```python
from build123d import *

# Parameters (mm, degrees)
SKETCH1_W           = 50
SKETCH1_H           = 80
BOSS_EXTRUDE1_DEPTH = 4.5
SKETCH2_R           = 0.5
CUT_EXTRUDE1_DEPTH  = 95.447075127
SKETCH3_W           = 2
SKETCH3_H           = 2.25
CUT_EXTRUDE2_DEPTH  = 95.447075127
SKETCH5_R           = 2.5
BOSS_EXTRUDE2_DEPTH = 2
SKETCH6_R           = 1.5
CUT_EXTRUDE3_DEPTH  = 95.563470748
FILLET1_R           = 4
SKETCH8_W           = 5.5
SKETCH8_H           = 30
CUT_EXTRUDE4_DEPTH  = 3


with BuildPart() as part:
    # Sketch1 → Boss-Extrude1 (new body)
    with BuildSketch(Plane(origin=(0, 0, 0), x_dir=(0, 1, 0), z_dir=(0, 0, 1))):
        with Locations((25, 40)):
            Rectangle(SKETCH1_W, SKETCH1_H)
    extrude(amount=BOSS_EXTRUDE1_DEPTH)

    # Sketch2 → Cut-Extrude1 (cut, through all)
    with BuildSketch(Plane.XY.offset(4.5)):
        with Locations((-45, 25)):
            Circle(SKETCH2_R)
    extrude(amount=-CUT_EXTRUDE1_DEPTH, mode=Mode.SUBTRACT)

    # Sketch3 → Cut-Extrude2 (cut, through all)
    with BuildSketch(Plane(origin=(-80, 0, 0), x_dir=(0, -1, 0), z_dir=(-1, 0, 0))):
        with Locations((-49, 1.125)):
            Rectangle(SKETCH3_W, SKETCH3_H)
        with Locations((-1, 1.125)):
            Rectangle(SKETCH3_W, SKETCH3_H)
    extrude(amount=-CUT_EXTRUDE2_DEPTH, mode=Mode.SUBTRACT)

    # Sketch5 → Boss-Extrude2 (add)
    with BuildSketch(Plane.XY.offset(4.5)):
        with Locations(Location((-45, 25, 0), (0, 0, 180))):
            Circle(SKETCH5_R)
    extrude(amount=BOSS_EXTRUDE2_DEPTH)

    # Sketch6 → Cut-Extrude3 (cut, through all)
    with BuildSketch(Plane.XY.offset(6.5)):
        with Locations((-45, 25)):
            Circle(SKETCH6_R)
    extrude(amount=-CUT_EXTRUDE3_DEPTH, mode=Mode.SUBTRACT)

    # Fillet1
    # the kernel refuses this fillet: 4 mm, written as the material it adds along each edge
    with BuildSketch(Plane(origin=(-45, 25, 4.5), x_dir=(-1, 0, 0), z_dir=(0, 1, 0))) as fillet1_piece_1:
        with BuildLine():
            CenterArc((5.964101615, 4), FILLET1_R, 210, 60)
            Line((2.5, 2), (2.430717968, 1.96))
            ThreePointArc((2.430717968, 1.96), (2.42, 1), (2.42, 0))
            Line((2.42, 0), (2.5, -0.08))
            Line((2.5, -0.08), (5.964101615, -0.08))
            Line((5.964101615, -0.08), (5.964101615, 0))
        make_face()
    revolve(axis=Axis((-45, 25, 4.5), (0, 0, 1)))

    # Sketch8 → Cut-Extrude4 (cut)
    with BuildSketch(Plane(origin=(0, 0, 0), x_dir=(1, 0, 0), z_dir=(0, 0, -1))):
        with Locations((-45, -35)):
            Rectangle(SKETCH8_W, SKETCH8_H)
    extrude(amount=-CUT_EXTRUDE4_DEPTH, mode=Mode.SUBTRACT)


solid = part.part
```
Verification items for the finished model (mm, model axes). A direction names the side the tool comes from. Give positions to 0.01 mm unless a question says otherwise; leave off trailing zeros. Order: outer loops, then holes, each group sorted by start corner. A loop starts at its lowest first (then second) coordinate and runs counter-clockwise, first axis right, second up. Notation, with made-up numbers: (-20, 82.25) -> (-14, 82.25) arc R26 ccw to (-14, 114.25) -> close; hole circle Ø1 at (73.25, 25.5). An arc over 180 degrees is marked (long way). One line per item, written item: value.
(1) Scan lines: line 1 along Y through (x, z) = (-45, 4); line 2 along Z through (x, y) = (-9, 14.5); line 3 along X through (y, z) = (35, 0.5). Record each from-to range of solid material in increasing order. Write a range as [from, to].
Final values:
line 1: [0, 23.5], [26.5, 50]
line 2: [0, 4.5]
line 3: [-80, -47.75], [-42.25, 0]
(2) Sectioned sample at B-B on y = 25. Record the cut outline in (x, z).
Final values:
outline: (-80, 0) -> (-47.75, 0) -> (-47.75, 3) -> (-46.5, 3) -> (-46.5, 6.5) -> (-47.5, 6.5) arc R4 cw to (-50.96, 4.5) -> (-80, 4.5) -> close; (-43.5, 3) -> (-42.25, 3) -> (-42.25, 0) -> (0, 0) -> (0, 4.5) -> (-39.04, 4.5) arc R4 cw to (-42.5, 6.5) -> (-43.5, 6.5) -> close
(3) Sectioned sample at A-A on x = -45. Record the cut outline in (y, z).
Final values:
outline: (0, 2.25) -> (2, 2.25) -> (2, 0) -> (20, 0) -> (20, 3) -> (23.5, 3) -> (23.5, 6.5) -> (22.5, 6.5) arc R4 cw to (19.04, 4.5) -> (0, 4.5) -> close; (26.5, 3) -> (50, 3) -> (50, 4.5) -> (30.96, 4.5) arc R4 cw to (27.5, 6.5) -> (26.5, 6.5) -> close
(4) Tool access check on faces 5 (the face through (-42.25, 35, 1)), 6 (the face through (-21, 49, 2.25)), 7 (the face through (-41, 1, 2.25)). Record the directions out of +Z, -Z, +X, -X, +Y, -Y that give a thin tool (end or side, any length) a straight path to the whole face; none if there is none.
Final values:
face 5: -Z, +Y
face 6: -Z, +X, -X, +Y
face 7: -Z, +X, -X, -Y
(5) Sectioned sample at D-D on x = -55. Record the cut outline in (y, z), then the cut area to 3 significant figures.
Final values:
outline: (0, 2.25) -> (2, 2.25) -> (2, 0) -> (48, 0) -> (48, 2.25) -> (50, 2.25) -> (50, 4.5) -> (0, 4.5) -> close
area: 216 mm^2
(6) Gauge pin test, flat ends, axial feed: pin 1 (8 mm diameter, centred on x = -67, y = 11.5, fed in from +Z); pin 2 (5 mm diameter, centred on x = -45, y = 25, fed in from -Z); pin 3 (1.6 mm diameter, centred on x = -16.5, y = 49, fed in from -Z). Record the tip position at first contact, or that the pin passes through.
Final values:
pin 1: z = 4.5
pin 2: z = 3
pin 3: z = 2.25
(7) Draft check along X on faces 1 (the face through (0, 25, 2)), 2 (the face through (-46.11, 26.01, 4.77)), 3 (the face through (-80, 25, 2)), 4 (the face through (-39, 50, 3)). Enter one of: pulls with the +X half, pulls with the -X half, needs draft (parallel to the pull), parting line crosses it, or undercut.
Final values:
face 1: pulls with the +X half
face 2: undercut
face 3: pulls with the -X half
face 4: needs draft
(8) Sectioned sample at C-C on z = 1.25. Record the cut outline in (x, y).
Final values:
outline: (-80, 2) -> (0, 2) -> (0, 48) -> (-42.25, 48) -> (-42.25, 20) -> (-47.75, 20) -> (-47.75, 48) -> (-80, 48) -> close
